```python
from build123d import *

# Parameters (mm, degrees)
BOSS_EXTRUDE1_DEPTH = 38.1
SKETCH2_W           = 31.75
SKETCH2_H           = 31.75
CUT_EXTRUDE1_DEPTH  = 198.452983021


with BuildPart() as part:
    # Sketch1 → Boss-Extrude1 (new body)
    with BuildSketch(Plane(origin=(0, 0, 0), x_dir=(0, 0, -1), z_dir=(1, 0, 0))):
        with BuildLine():
            Line((0, 189.959102187), (0, 0))
            Line((0, 0), (38.1, 0))
            Line((38.1, 0), (38.1, 189.959102187))
            ThreePointArc((38.1, 189.959102187), (19.05, 180.63972), (0, 189.959102187))
        make_face()
    extrude(amount=BOSS_EXTRUDE1_DEPTH)

    # Sketch2 → Cut-Extrude1 (cut, through all)
    with BuildSketch(Plane.XZ):
        with Locations((19.05, -19.05)):
            Rectangle(SKETCH2_W, SKETCH2_H)
    extrude(amount=-CUT_EXTRUDE1_DEPTH, mode=Mode.SUBTRACT)


solid = part.part
```
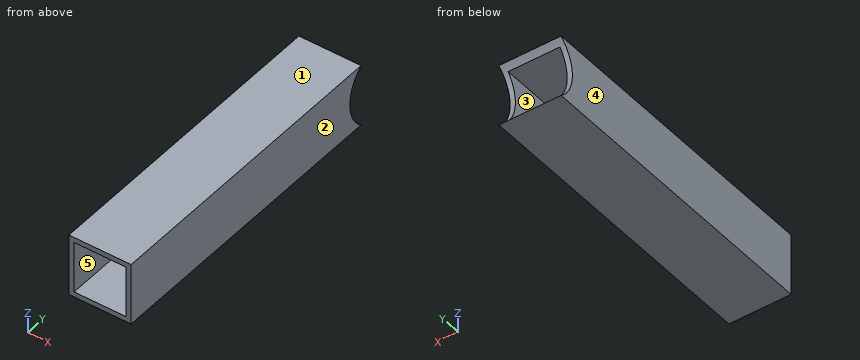
The listing builds one solid part. Answer for the finished solid, in the listing's coordinates (mm). Face numbers are marked on the shaded views. A direction names the side the tool comes from. Coordinates: 2 decimals unless noted, no trailing zeros. Loops run counter-clockwise (first coordinate to the right, second up) from the corner with the lowest first, then second, coordinate; pieces in that order, holes last. Notation, with made-up numbers: (-16, 20.5) - (10, 20.5) arc R4 cw to (10, 25.5) - close; hole circle Ø8 at (66.25, 1). An arc over 180 degrees is marked (long way). Use a Markdown table: item, result. Add a question column.
1) The mould has two halves that part along X. Classify the marked faces 1, 2 and 3: released by +X, released by -X, zero draft, split by the parting line, or undercut.
2) The part is cut by section C-C, the plane z = -24. Give the vertices of the cut face in (x, y) (3 decimals).
3) Find the intervals of material crossed by line 1 (X direction, y = 104, z = -6.5) (3 decimals); line 2 (Z direction, x = 7, y = 138) (3 decimals); line 3 (Y direction, x = 3, z = -3), in increasing order.
4) For the marked faces 4 and 5, determine the directions among +Z, -Z, +X, -X, +Y, -Y from which every point of the face is accessible in a straight line to the end or side of a thin tool.
5) The part is cut by section B-B, the plane y = 172. Give the vertices of the cut face in (x, z) (3 decimals).
6) The part is cut by section A-A, the plane x = 25. Give the vertices of the cut face in (y, z) (3 decimals), and give its area (3 significant figures).
Here are the results:
| question | item | result |
|---|---|---|
| 1 | face 1 | zero draft |
| 1 | face 2 | released by +X |
| 1 | face 3 | undercut |
| 2 | outline | (0, 0) - (3.175, 0) - (3.175, 181.153) - (0, 181.153) - close; (34.925, 0) - (38.1, 0) - (38.1, 181.153) - (34.925, 181.153) - close |
| 3 | line 1 | x = 0 to 3.175, 34.925 to 38.1 |
| 3 | line 2 | z = -38.1 to -34.925, -3.175 to 0 |
| 3 | line 3 | y = 0 to 186.75 |
| 4 | face 4 | +Z, -Z, -X, +Y, -Y |
| 4 | face 5 | +Y, -Y |
| 5 | outline | (0, -38.1) - (38.1, -38.1) - (38.1, 0) - (0, 0) - close; hole (3.175, -34.925) - (34.925, -34.925) - (34.925, -3.175) - (3.175, -3.175) - close |
| 6 | outline | (0, -38.1) - (189.959, -38.1) arc R24.13 cw to (186.597, -34.925) - (0, -34.925) - close; (0, -3.175) - (186.597, -3.175) arc R24.13 cw to (189.959, 0) - (0, 0) - close |
| 6 | area | 1,190 mm^2 |
